Geometry check sheet. Reference: the model listing, model coordinates, mm. A direction names the side the tool comes from. Round coordinates to 2 decimals unless told otherwise and drop trailing zeros. Write each loop counter-clockwise with the first axis right and the second up, starting at its lowest first coordinate (ties: lowest second). Pieces come first, ordered by that corner, then holes. Notation, with made-up numbers: (81.5, 60) -> (123.5, 60) arc R19 ccw to (123.5, 64) -> close; hole circle Ø3 at (59.25, -13.75). An arc over 180 degrees is marked (long way). Return JSON: item names as keys, results as strings. Group by question number.
from build123d import *

# Parameters (mm, degrees)
EXTRUDE_1_DEPTH = 214
EXTRUDE_2_DEPTH = 23
EXTRUDE_3_DEPTH = 28
FILLET_1_R      = 5
SKETCH_4_W      = 244
SKETCH_4_H      = 105
SKETCH_4_R      = 3.25
EXTRUDE_4_DEPTH = 1
FILLET_2_R      = 5
SKETCH_5_W      = 120
SKETCH_5_H      = 64
EXTRUDE_5_DEPTH = 40


with BuildPart() as part:
    # Эскиз1 → Бобышка-Вытянуть1 (new body)
    with BuildSketch(Plane(origin=(0, 0, 0), x_dir=(0, 0, -1), z_dir=(1, 0, 0))):
        with BuildLine():
            Line((-60, 0), (60, 0))
            Line((60, 0), (60, 64))
            ThreePointArc((60, 64), (32.877245052, 71.055175037), (5, 73.932420089))
            Line((5, 73.932420089), (5, 64))
            Line((5, 64), (-14, 64))
            Line((-14, 64), (-14, 73.469509676))
            ThreePointArc((-14, 73.469509676), (-37.301714483, 70.200392098), (-60, 64))
            Line((-60, 64), (-60, 0))
        make_face()
    extrude(amount=EXTRUDE_1_DEPTH)

    # Эскиз2 → Бобышка-Вытянуть2 (add)
    with BuildSketch(Plane.ZY):
        Polygon((-19, 32), (-25.25, 42.825317547), (-37.75, 42.825317547), (-44, 32), (-37.75, 21.174682453), (-25.25, 21.174682453), align=None)
    extrude(amount=EXTRUDE_2_DEPTH)

    # Эскиз2<3> → Бобышка-Вытянуть3 (add)
    with BuildSketch(Plane.ZY):
        Polygon((50, 32), (41, 47.588457268), (23, 47.588457268), (14, 32), (23, 16.411542732), (41, 16.411542732), align=None)
    extrude(amount=EXTRUDE_3_DEPTH)

    # Скругление1
    fillet_1_edges = [part.edges().sort_by_distance(p)[0] for p in [
        (-23, 42.825317547, -31.5),
        (-23, 37.412658774, -40.875),
        (-23, 26.587341226, -40.875),
        (-23, 21.174682453, -31.5),
        (-23, 26.587341226, -22.125),
        (-23, 37.412658774, -22.125),
        (-28, 39.794228634, 45.5),
        (-28, 47.588457268, 32),
        (-28, 39.794228634, 18.5),
        (-28, 24.205771366, 18.5),
        (-28, 16.411542732, 32),
        (-28, 24.205771366, 45.5),
    ]]
    fillet(fillet_1_edges, radius=FILLET_1_R)

    # Эскиз4 → Бобышка-Вытянуть4 (add)
    with BuildSketch(Plane.XZ):
        with Locations((107, 0)):
            Rectangle(SKETCH_4_W, SKETCH_4_H)
        with Locations((221.5, 0)):
            Circle(SKETCH_4_R, mode=Mode.SUBTRACT)
        with Locations((-7.5, 0)):
            Circle(SKETCH_4_R, mode=Mode.SUBTRACT)
        with BuildLine():
            Line((224.75, 37.75), (224.75, 17.25))
            ThreePointArc((224.75, 17.25), (221.5, 14), (218.25, 17.25))
            Line((218.25, 17.25), (218.25, 37.75))
            ThreePointArc((218.25, 37.75), (221.5, 41), (224.75, 37.75))
        make_face(mode=Mode.SUBTRACT)
        with BuildLine():
            Line((224.75, -37.75), (224.75, -17.25))
            ThreePointArc((224.75, -17.25), (221.5, -14), (218.25, -17.25))
            Line((218.25, -17.25), (218.25, -37.75))
            ThreePointArc((218.25, -37.75), (221.5, -41), (224.75, -37.75))
        make_face(mode=Mode.SUBTRACT)
        with BuildLine():
            Line((-10.75, 37.75), (-10.75, 17.25))
            ThreePointArc((-10.75, 17.25), (-7.5, 14), (-4.25, 17.25))
            Line((-4.25, 17.25), (-4.25, 37.75))
            ThreePointArc((-4.25, 37.75), (-7.5, 41), (-10.75, 37.75))
        make_face(mode=Mode.SUBTRACT)
        with BuildLine():
            Line((-10.75, -37.75), (-10.75, -17.25))
            ThreePointArc((-10.75, -17.25), (-7.5, -14), (-4.25, -17.25))
            Line((-4.25, -17.25), (-4.25, -37.75))
            ThreePointArc((-4.25, -37.75), (-7.5, -41), (-10.75, -37.75))
        make_face(mode=Mode.SUBTRACT)
    extrude(amount=-EXTRUDE_4_DEPTH)

    # Скругление2
    fillet_2_edges = [part.edges().sort_by_distance(p)[0] for p in [
        (229, 0.5, -52.5),
        (-15, 0.5, -52.5),
        (-15, 0.5, 52.5),
        (229, 0.5, 52.5),
    ]]
    fillet(fillet_2_edges, radius=FILLET_2_R)

    # Эскиз5 → Бобышка-Вытянуть5 (add)
    with BuildSketch(Plane.ZY.offset(28)):
        with Locations((0, 32)):
            Rectangle(SKETCH_5_W, SKETCH_5_H)
    extrude(amount=EXTRUDE_5_DEPTH)


solid = part.part
1) Go/stop test with flat-tipped pins: P1, Ø4, axis at x = 15, z = -32.5, coming from the -Y side; P2, Ø1.1, axis at x = -7, y = 0.5, coming from the +Z side; P3, Ø20, axis at x = -10.5, z = 34, coming from the +Y side; P4, Ø2, axis at x = 14.5, z = -26, coming from the +Y side. Record where each tip stops, or that it passes through.
2) Material ranges on probe 1 along Z at (x, y) = (221.5, 0.25); probe 2 along X at (y, z) = (48, -39.5); probe 3 along X at (y, z) = (34, -31), recorded low to high. Write a range as [from, to].
3) Sectioned sample at B-B on x = -48. Enter the section's corners in (y, z).
4) Tool access check on faces 5 (the face through (-11.34, 39.69, 45.56)), 6 (the face through (106, 64, 4)), 7 (the face through (0, 37, 1)), 8 (the face through (-9, 21.175, -32)). Record the directions out of +Z, -Z, +X, -X, +Y, -Y that give a thin tool (end or side, any length) a straight path to the whole face; none if there is none.
5) Sectioned sample at A-A on x = 4. Enter the section's corners in (y, z).
6) Mould release check, pull along Z, two halves, no side actions. Record for faces 1 (the face through (227.57, 0.51, -51)), 2 (the face through (-11.34, 39.9, 18.56)), 3 (the face through (-11, 47.588, 32)), 4 (the face through (-21.496, 36.776, -23.404)): +Z half, -Z half, draft (parallel to the pull), parting line (faces both ways), or undercut.
Evaluation:
{
 "1": {"P1": "stops at y = 0", "P2": "stops at z = 52.5", "P3": "stops at y = 47.59", "P4": "stops at y = 72.3"},
 "2": {"probe 1": "z = [-52.5, -41], [-14, -3.25], [3.25, 14], [41, 52.5]", "probe 2": "x = [-68, -28], [0, 214]", "probe 3": "x = [-68, -28], [-23, 214]"},
 "3": {"outline": "(0, -60) -> (64, -60) -> (64, 60) -> (0, 60) -> close"},
 "4": {"face 5": "+Z, +Y", "face 6": "+X, -X, +Y", "face 7": "none", "face 8": "-Z"},
 "5": {"outline": "(0, -60) -> (64, -60) arc R185 ccw to (73.93, -5) -> (64, -5) -> (64, 14) -> (73.47, 14) arc R185 ccw to (64, 60) -> (0, 60) -> close"},
 "6": {"face 1": "-Z half", "face 2": "undercut", "face 3": "draft", "face 4": "undercut"}
}
